from build123d import *

# Parameters (mm, degrees)
SKETCH1_W           = 60
SKETCH1_H           = 60
SKETCH1_R           = 15
BOSS_EXTRUDE1_DEPTH = 10
SKETCH2_R           = 3
CUT_EXTRUDE1_DEPTH  = 10
SKETCH3_R           = 6.5
CUT_EXTRUDE2_DEPTH  = 5
SKETCH4_R           = 3
CUT_EXTRUDE3_DEPTH  = 10


with BuildPart() as part:
    # Sketch1 → Boss-Extrude1 (new body)
    with BuildSketch(Plane(origin=(0, 0, 0), x_dir=(1, 0, 0), z_dir=(0, 1, 0))):
        with Locations((30, 30)):
            Rectangle(SKETCH1_W, SKETCH1_H)
        with Locations(Location((30, 30, 0), (0, 0, 270))):
            Circle(SKETCH1_R, mode=Mode.SUBTRACT)
    extrude(amount=BOSS_EXTRUDE1_DEPTH)

    # Sketch2 → Cut-Extrude1 (cut)
    with BuildSketch(Plane(origin=(0, 10, 0), x_dir=(1, 0, 0), z_dir=(0, 1, 0))):
        with Locations(Location((30, 50, 0), (0, 0, 270))):
            Circle(SKETCH2_R)
        with Locations(Location((50, 30, 0), (0, 0, 270))):
            Circle(SKETCH2_R)
        with Locations(Location((30, 10, 0), (0, 0, 270))):
            Circle(SKETCH2_R)
        with Locations(Location((10, 30, 0), (0, 0, 270))):
            Circle(SKETCH2_R)
    extrude(amount=-CUT_EXTRUDE1_DEPTH, mode=Mode.SUBTRACT)

    # Sketch3 → Cut-Extrude2 (cut)
    with BuildSketch(Plane(origin=(0, 10, 0), x_dir=(1, 0, 0), z_dir=(0, 1, 0))):
        with Locations((30, 50)):
            Circle(SKETCH3_R)
        with Locations((50, 30)):
            Circle(SKETCH3_R)
        with Locations((30, 10)):
            Circle(SKETCH3_R)
        with Locations((10, 30)):
            Circle(SKETCH3_R)
    extrude(amount=-CUT_EXTRUDE2_DEPTH, mode=Mode.SUBTRACT)

    # Sketch4 → Cut-Extrude3 (cut)
    with BuildSketch(Plane.XZ):
        with Locations(Location((5, -5, 0), (0, 0, 270))):
            Circle(SKETCH4_R)
        with Locations(Location((55, -5, 0), (0, 0, 270))):
            Circle(SKETCH4_R)
        with Locations(Location((55, -55, 0), (0, 0, 270))):
            Circle(SKETCH4_R)
        with Locations(Location((5, -55, 0), (0, 0, 270))):
            Circle(SKETCH4_R)
    extrude(amount=-CUT_EXTRUDE3_DEPTH, mode=Mode.SUBTRACT)


solid = part.part
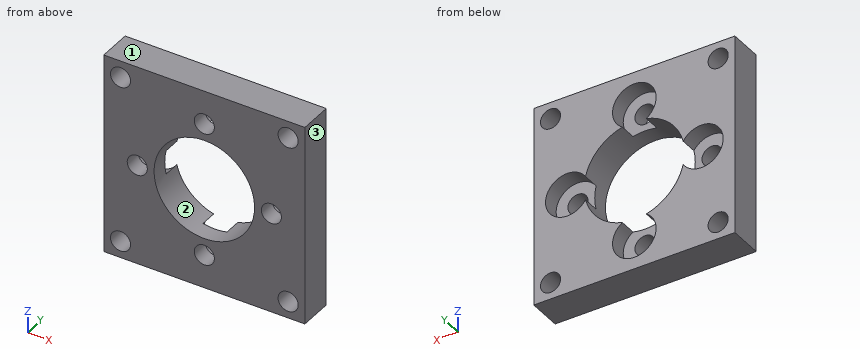
CAD build for the part. Positions are in the model's coordinates, mm. Face numbers are marked on the shaded views. Give positions to 0.01 mm unless a question says otherwise; leave off trailing zeros. Write each loop counter-clockwise with the first axis right and the second up, starting at its lowest first coordinate (ties: lowest second). Pieces come first, ordered by that corner, then holes. Notation, with made-up numbers: (1.5, 4) - (24.5, 4) arc R19 ccw to (24.5, 21) - close; hole circle Ø3 at (79, 82). An arc over 180 degrees is marked (long way). Put each result on its own line as item: value.
(1) Saw through at B-B (x = 50). List the corners of the cut face in (y, z), then the cut area to 3 significant figures.
Working result:
outline: (0, -60) - (10, -60) - (10, -36.5) - (5, -36.5) - (5, -33) - (0, -33) - close; (0, -27) - (5, -27) - (5, -23.5) - (10, -23.5) - (10, 0) - (0, 0) - close
area: 505 mm^2
(2) Saw through at C-C (y = 2). Count the separate pieces of the cut face and the enclosed holes in it, then the cut area to 3 significant figures.
Working result:
separate pieces: 1
enclosed holes: 9
area: 2,670 mm^2
(3) Saw through at D-D (x = 30). List the corners of the cut face in (y, z).
Working result:
outline: (0, -60) - (10, -60) - (10, -56.5) - (5, -56.5) - (5, -53) - (0, -53) - close; (0, -47) - (5, -47) - (5, -45) - (0, -45) - close; (0, -15) - (5, -15) - (5, -13) - (0, -13) - close; (0, -7) - (5, -7) - (5, -3.5) - (10, -3.5) - (10, 0) - (0, 0) - close
(4) Pull direction X, two halves, no side cores. Call the marked faces 1, 2 and 3: released by +X, released by -X, zero draft, split by the parting line, or undercut.
Working result:
face 1: zero draft
face 2: undercut
face 3: released by +X
(5) Wall check: L1, parallel to X at y = 3.25, z = -55; L2, parallel to X at y = 8.85, z = -10; L3, parallel to X at y = 6.25, z = -30. Give the ranges that are in metal, low to high.
Working result:
L1: 0 to 2, 8 to 52, 58 to 60
L2: 0 to 23.5, 36.5 to 60
L3: 0 to 3.5, 56.5 to 60
(6) Saw through at A-A (z = -30). List the corners of the cut face in (x, y).
Working result:
outline: (0, 0) - (7, 0) - (7, 5) - (3.5, 5) - (3.5, 10) - (0, 10) - close; (13, 0) - (15, 0) - (15, 5) - (13, 5) - close; (45, 0) - (47, 0) - (47, 5) - (45, 5) - close; (53, 0) - (60, 0) - (60, 10) - (56.5, 10) - (56.5, 5) - (53, 5) - close
(7) Drop flat-ended pins along their axis: pin 1 Ø7 at (x, z) = (30, -50) entering from +Y; pin 2 Ø10 at (x, z) = (33.5, -17) entering from -Y; pin 3 Ø5 at (x, z) = (5, -55) entering from +Y. Give the stop position or say it passes through.
Working result:
pin 1: y = 5
pin 2: y = 0
pin 3: through
